```python
from build123d import *

# Parameters (mm, degrees)
F0_W     = 2.5
F0_H     = 4.5
F1_DEPTH = 1.25


with BuildPart() as f1:
    # F0 (on Top) → F1 (new body)
    with BuildSketch(Plane.XY):
        with BuildLine():
            Line((8.2, 1.5), (6.837397, 1.5))
            ThreePointArc((6.837397, 1.5), (0, 7), (-6.837397, 1.5))
            Line((-6.837397, 1.5), (-8.2, 1.5))
            Line((-8.2, 1.5), (-8.2, -1.5))
            Line((-8.2, -1.5), (-6.837397, -1.5))
            ThreePointArc((-6.837397, -1.5), (0, -7), (6.837397, -1.5))
            Line((6.837397, -1.5), (8.2, -1.5))
            Line((8.2, -1.5), (8.2, 1.5))
        make_face()
        with Locations((-3.8, 0)):
            Rectangle(F0_W, F0_H, mode=Mode.SUBTRACT)
        with Locations((3.8, 0)):
            Rectangle(F0_W, F0_H, mode=Mode.SUBTRACT)
    extrude(amount=F1_DEPTH)


solid = f1.part
```
Check sheet for the modelled part. Datum: model origin and axes. Units: mm. A direction names the side the tool comes from. Coordinates: 2 decimals unless noted, no trailing zeros. Order: outer loops, then holes, each group sorted by start corner. A loop starts at its lowest first (then second) coordinate and runs counter-clockwise, first axis right, second up. Notation, with made-up numbers: M -28.5,17 L 16.5,17 A31 ccw 16.5,51 Z; hole C -13.5,38.5 d7. An arc over 180 degrees is marked long. Write each question's results on one line, items separated by ' | '. Start each with the question number.
1. Access from +Z, -Z, +X, -X, +Y, -Y to the whole of each face (thin tool, end or side, straight path). Record for faces 1 (the face through (5.05, 0, 1)), 2 (the face through (-8, -1.5, 1)), 3 (the face through (8, -1.5, 1)).
2. Mould release check, pull along Y, two halves, no side actions. Record for faces 4 (the face through (4, -2.25, 1)), 5 (the face through (0, -7, 1)), 6 (the face through (8, 1.5, 1)), 7 (the face through (4, 2.25, 1)): +Y half, -Y half, draft (parallel to the pull), parting line (faces both ways), or undercut.
3. Cross-section at D-D on y = 2. Record the cut outline in (x, z).
4. Cross-section at A-A on y = -1.25. Record the cut outline in (x, z), and give its area (4 significant figures).
5. Material ranges on probe 1 along X at (y, z) = (0, 0.55); probe 2 along X at (y, z) = (2, 0.1); probe 3 along Y at (x, z) = (1.5, 0.45), recorded low to high.
6. Cross-section at C-C on x = -4.75. Record the cut outline in (y, z), and give its area (3 significant figures).
7. Cross-section at B-B on z = 0.9. Record the cut outline in (x, y), and give its area (3 significant figures).
Checks:
1) face 1: +Z, -Z | face 2: +Z, -Z, -X, -Y | face 3: +Z, -Z, +X, -Y
2) face 4: undercut | face 5: -Y half | face 6: +Y half | face 7: undercut
3) outline: M -6.71,0 L -5.05,0 L -5.05,1.25 L -6.71,1.25 Z; M -2.55,0 L 2.55,0 L 2.55,1.25 L -2.55,1.25 Z; M 5.05,0 L 6.71,0 L 6.71,1.25 L 5.05,1.25 Z
4) outline: M -8.2,0 L -5.05,0 L -5.05,1.25 L -8.2,1.25 Z; M -2.55,0 L 2.55,0 L 2.55,1.25 L -2.55,1.25 Z; M 5.05,0 L 8.2,0 L 8.2,1.25 L 5.05,1.25 Z | area: 14.25 mm²
5) probe 1: x = -8.2 to -5.05, -2.55 to 2.55, 5.05 to 8.2 | probe 2: x = -6.71 to -5.05, -2.55 to 2.55, 5.05 to 6.71 | probe 3: y = -6.84 to 6.84
6) outline: M -5.14,0 L -2.25,0 L -2.25,1.25 L -5.14,1.25 Z; M 2.25,0 L 5.14,0 L 5.14,1.25 L 2.25,1.25 Z | area: 7.23 mm²
7) outline: M -8.2,-1.5 L -6.84,-1.5 A7 ccw 6.84,-1.5 L 8.2,-1.5 L 8.2,1.5 L 6.84,1.5 A7 ccw -6.84,1.5 L -8.2,1.5 Z; hole M -5.05,-2.25 L -2.55,-2.25 L -2.55,2.25 L -5.05,2.25 Z; hole M 2.55,-2.25 L 5.05,-2.25 L 5.05,2.25 L 2.55,2.25 Z | area: 139 mm²
